from build123d import *

# Parameters (mm, degrees)
F0_R          = 10
F0_R_2        = 7.525
F1_DEPTH      = 2
F1_TAPER      = -10
F1_DEPTH_BACK = 2
F1_TAPER_BACK = -10
F0_R_3        = 7.5
F0_R_4        = 5
F2_DEPTH      = 2
F2_TAPER      = -10
F2_DEPTH_BACK = 2
F2_TAPER_BACK = -10
F3_R          = 12.6754374972
F3_R_2        = 10
F4_DEPTH      = 2
F4_DEPTH_BACK = 2
F5_R          = 5
F5_R_2        = 1.8774489935
F6_DEPTH      = 2
F6_DEPTH_BACK = 2


with BuildPart() as f1:
    # F0 (on Top) → F1 (new body, two sides)
    with BuildSketch(Plane.XY) as f1_sk:
        Circle(F0_R)
        Circle(F0_R_2, mode=Mode.SUBTRACT)
    extrude(amount=F1_DEPTH, taper=F1_TAPER)
    extrude(f1_sk.sketch, amount=-F1_DEPTH_BACK, taper=F1_TAPER_BACK)

    # F0 (on Top) → F2 (join, two sides)
    with BuildSketch(Plane.XY) as f2_sk:
        Circle(F0_R_3)
        Circle(F0_R_4, mode=Mode.SUBTRACT)
    extrude(amount=F2_DEPTH, taper=F2_TAPER)
    extrude(f2_sk.sketch, amount=-F2_DEPTH_BACK, taper=F2_TAPER_BACK)

    # F3 (on Top) → F4 (cut, two sides)
    with BuildSketch(Plane.XY) as f4_sk:
        Circle(F3_R)
        Circle(F3_R_2, mode=Mode.SUBTRACT)
    extrude(amount=-F4_DEPTH, mode=Mode.SUBTRACT)
    extrude(f4_sk.sketch, amount=F4_DEPTH_BACK, mode=Mode.SUBTRACT)

    # F5 (on Top) → F6 (cut, two sides)
    with BuildSketch(Plane.XY) as f6_sk:
        Circle(F5_R)
        Circle(F5_R_2, mode=Mode.SUBTRACT)
    extrude(amount=-F6_DEPTH, mode=Mode.SUBTRACT)
    extrude(f6_sk.sketch, amount=F6_DEPTH_BACK, mode=Mode.SUBTRACT)


solid = f1.part
The listing builds one solid part. Answer for the finished solid, in the listing's coordinates (mm). Give positions to 0.01 mm unless a question says otherwise; leave off trailing zeros. Order: outer loops, then holes, each group sorted by start corner. A loop starts at its lowest first (then second) coordinate and runs counter-clockwise, first axis right, second up. Notation, with made-up numbers: (62.25, -18) - (96.25, -18) arc R17 ccw to (96.25, 8) - close; hole circle Ø1 at (31.25, 49.5). An arc over 180 degrees is marked (long way). One line per item, written item: value. Start each with the question number.
1) Given pin 1 Ø9 at (x, y) = (0, 0) entering from +Z; pin 2 Ø1 at (y, z) = (-8, -1.5) entering from -X, each flat-ended and moving along its own axis, determine where each tip first touches the part or whether it passes through.
2) A cutting plane is placed at A-A on x = 0. State how many separate pieces and enclosed holes the cut face has, then the cut area to 3 significant figures.
3) A cutting plane is placed at C-C on z = 1.1. Give the vertices of the cut face in (x, y).
4) Find the intervals of material crossed by L1, parallel to Y at x = 0, z = 0.95; L2, parallel to Y at x = -2.5, z = -0.8; L3, parallel to X at y = 0.5, z = -0.8, in increasing order.
Answer sheet:
1. pin 1: passes through
1. pin 2: stops at x = -6.61
2. separate pieces: 2
2. enclosed holes: 2
2. area: 40.0 mm2
3. outline: circle Ø20 at (0, 0); hole circle Ø10 at (0, 0)
4. L1: y = -10 to -5, 5 to 10
4. L2: y = -9.68 to -4.33, 4.33 to 9.68
4. L3: x = -9.99 to -4.97, 4.97 to 9.99
